Geometry check sheet. Reference: the model listing, model coordinates, mm. Give positions to 0.01 mm unless a question says otherwise; leave off trailing zeros. Use one line per item in the form item = value. Start each with the question number.
Autodesk Inventor part; units mm, degrees
ref_plane "YZ Plane" through (0, 0, 0) normal (1, 0, 0) x (0, 1, 0)
ref_plane "XZ Plane" through (0, 0, 0) normal (0, 1, 0) x (-1, 0, 0)
ref_plane "XY Plane" through (0, 0, 0) normal (0, 0, 1) x (1, 0, 0)
sketch "Sketch1" plane through (0, 0, 0) normal (0, 1, 0) x (-1, 0, 0)
  circle A0 centre (19.05, -19.05) radius 3.3274
  circle A1 centre (19.05, -57.15) radius 3.3274
  circle A2 centre (19.05, -95.25) radius 3.3274
  line L0 (0, 0) -> (15.0114, 0)
  line L1 (15.0114, 0) -> (15.0114, -4.2672)
  line L2 (15.0114, -4.2672) -> (8.001, -4.2672)
  line L3 (38.1, 0) -> (23.0886, 0)
  line L4 (23.0886, 0) -> (23.0886, -4.2672)
  line L5 (23.0886, -4.2672) -> (30.099, -4.2672)
  line L6 (8.001, -4.2672) -> (15.0114, -11.9888)
  line L7 (30.099, -4.2672) -> (23.0886, -11.9888)
  line L8 (23.0886, -11.9888) -> (15.0114, -11.9888)
  line L9 (38.1, 0) -> (38.1, -15.0114)
  line L10 (38.1, -15.0114) -> (33.8328, -15.0114)
  line L11 (33.8328, -15.0114) -> (33.8328, -8.001)
  line L12 (26.1112, -15.0114) -> (26.1112, -25.8654)
  line L13 (33.8328, -8.001) -> (26.1112, -15.0114)
  line L14 (38.1, -24.6888) -> (33.8328, -24.6888)
  line L15 (33.8328, -24.6888) -> (33.8328, -31.6992)
  line L16 (33.8328, -31.6992) -> (26.1112, -25.8654)
  line L17 (38.1, -114.3) -> (38.1, -99.2886)
  line L18 (38.1, -99.2886) -> (33.8328, -99.2886)
  line L19 (33.8328, -99.2886) -> (33.8328, -106.299)
  line L20 (38.1, -114.3) -> (23.0886, -114.3)
  line L21 (23.0886, -114.3) -> (23.0886, -110.0328)
  line L22 (23.0886, -110.0328) -> (30.099, -110.0328)
  line L23 (0, -114.3) -> (15.0114, -114.3)
  line L24 (15.0114, -114.3) -> (15.0114, -110.0328)
  line L25 (15.0114, -110.0328) -> (8.001, -110.0328)
  line L26 (23.0886, -102.3112) -> (15.0114, -102.3112)
  line L27 (23.0886, -102.3112) -> (30.099, -110.0328)
  line L28 (15.0114, -102.3112) -> (8.001, -110.0328)
  line L29 (38.1, -24.6888) -> (38.1, -54.1528)
  line L30 (38.1, -54.1528) -> (33.8328, -54.1528)
  line L31 (33.8328, -54.1528) -> (33.8328, -47.1424)
  line L32 (26.1112, -54.6354) -> (26.1112, -62.7126)
  line L33 (33.8328, -47.1424) -> (26.1112, -54.6354)
  line L34 (38.1, -62.7126) -> (33.8328, -62.7126)
  line L35 (33.8328, -62.7126) -> (33.8328, -69.723)
  line L36 (33.8328, -69.723) -> (26.1112, -62.7126)
  line L37 (38.1, -91.9226) -> (33.8328, -91.9226)
  line L38 (33.8328, -91.9226) -> (33.8328, -84.9122)
  line L39 (38.1, -62.7126) -> (38.1, -91.9226)
  line L40 (28.0178, -91.9226) -> (28.0178, -99.2886)
  line L41 (28.0178, -99.2886) -> (33.8328, -106.299)
  line L42 (33.8328, -84.9122) -> (28.0178, -91.9226)
  line L43 (11.9888, -54.6354) -> (11.9888, -62.7126)
  line L44 (11.9888, -93.3774) -> (11.9888, -99.2886)
  line L45 (0, 0) -> (0, -15.0114)
  line L46 (0, -15.0114) -> (4.2672, -15.0114)
  line L47 (4.2672, -15.0114) -> (4.2672, -8.001)
  line L48 (11.9888, -15.7226) -> (11.9888, -25.8654)
  line L49 (4.2672, -8.001) -> (11.9888, -15.7226)
  line L50 (0, -114.3) -> (0, -99.2886)
  line L51 (0, -99.2886) -> (4.2672, -99.2886)
  line L52 (4.2672, -99.2886) -> (4.2672, -106.299)
  line L53 (4.2672, -106.299) -> (11.9888, -99.2886)
  line L54 (0, -63.9406) -> (0, -93.1506)
  line L55 (0, -93.1506) -> (4.2672, -93.1506)
  line L56 (4.2672, -93.1506) -> (4.2672, -86.1402)
  line L57 (4.2672, -86.1402) -> (11.9888, -93.3774)
  line L58 (0, -63.9406) -> (4.2672, -63.9406)
  line L59 (4.2672, -63.9406) -> (4.2672, -70.951)
  line L60 (4.2672, -70.951) -> (11.9888, -62.7126)
  line L61 (0, -55.2632) -> (0, -24.6888)
  line L62 (0, -24.6888) -> (4.5476, -24.6888)
  line L63 (4.5476, -24.6888) -> (4.5476, -31.6992)
  line L64 (4.5476, -31.6992) -> (11.9888, -25.8654)
  line L65 (0, -55.2632) -> (4.2672, -55.2632)
  line L66 (4.2672, -55.2632) -> (4.2672, -48.2528)
  line L67 (4.2672, -48.2528) -> (11.9888, -54.6354)
  dimension "d0" = 38.1
  dimension "d1" = 114.3
  dimension "d2" = 6.6548
  dimension "d3" = 6.6548
  dimension "d4" = 6.6548
  dimension "d11" = 15.0114
  dimension "d12" = 4.2672
  dimension "d14" = 15.0114
  dimension "d15" = 7.0104
  dimension "d19" = 15.0114
  dimension "d20" = 4.2672
  dimension "d21" = 7.0104
  dimension "d22" = 11.9888
  dimension "d23" = 4.2672
  dimension "d24" = 7.0104
  dimension "d25" = 9.6774
  dimension "d26" = 15.0114
  dimension "d27" = 7.0104
  dimension "d28" = 15.0114
  dimension "d29" = 4.2672
  dimension "d30" = 7.0104
  dimension "d31" = 15.0114
  dimension "d32" = 7.0104
  dimension "d33" = 11.9888
  dimension "d34" = 29.464
  dimension "d35" = 7.0104
  dimension "d36" = 8.0772
  dimension "d37" = 11.9888
  dimension "d38" = 7.0104
  dimension "d39" = 7.0104
  dimension "d40" = 15.0114
  dimension "d41" = 4.2672
  dimension "d42" = 7.0104
  dimension "d43" = 11.9888
  dimension "d44" = 11.9888
  dimension "d45" = 11.9888
  dimension "d46" = 15.0114
  dimension "d47" = 4.2672
  dimension "d48" = 7.0104
  dimension "d49" = 7.0104
  dimension "d50" = 4.2672
  dimension "d51" = 7.0104
  dimension "d52" = 29.21
  dimension "d53" = 29.21
  dimension "d54" = 7.0104
  dimension "d55" = 4.2672
  dimension "d56" = 7.0104
extrude "Extrusion1" add sketch "Sketch1" along normal blind 762
properties part number "1545rail_30inch"
(1) Sectioned sample at A-A, the plane y = 304.5. State how many separate pieces and enclosed holes the cut face has, plus the area to 3 significant figures.
(2) Depth check by flat-ended pin: pin 1 (6.5 mm diameter, centred on x = -19, y = 459.5, fed in from +Z); pin 2 (1 mm diameter, centred on x = -19.5, y = 609, fed in from -Z). Enter the tip coordinate at first touch or a pass-through.
(3) Thickness scan on probe 1 along Z at (x, y) = (-19, 183); probe 2 along X at (y, z) = (486, -57); probe 3 along X at (y, z) = (614.5, -102.5). Record the ranges inside material, lowest first. Write a range as [from, to].
Numbers:
q1.separate_pieces = 1
q1.enclosed_holes = 3
q1.area = 3,050 mm2
q2.pin_1 = -11.99
q2.pin_2 = -102.31
q3.probe_1 = [-102.31, -98.58], [-91.92, -60.48], [-53.82, -22.38], [-15.72, -11.99]
q3.probe_2 = [-26.11, -22.37], [-15.73, -11.99]
q3.probe_3 = [-38.1, -33.83], [-30.68, -23.26], [-14.84, -8.45], [-4.27, 0]
